Autodesk Inventor part; units mm, degrees
ref_plane "Work Plane19" through (16.25, 10, -160.125) normal (0, 0.3947, -0.9188) x (1, 0, 0)
ref_plane "Work Plane21" through (16.25, 10, -160.125) normal (0, 0.9118, 0.4107) x (1, 0, 0)
ref_plane "Work Plane22" through (16.25, 101.1762, -119.0531) normal (0, 0.9118, 0.4107) x (1, 0, 0)
sketch "Sketch1" plane through (0, 0, 0) normal (0, 1, 0) x (-1, 0, 0)
  circle A0 centre (0, 0) radius 135
  circle A1 centre (0, 0) radius 115
  circle A2 centre (0, 0) radius 112.0375
  circle A3 centre (0, 0) radius 9.5
  circle A4 centre (0, 0) radius 125
  circle A5 centre (0, -125) radius 2.75
  circle A6 centre (73.4732, -101.1271) radius 2.75
  circle A7 centre (118.8821, -38.6271) radius 2.75
  circle A8 centre (118.8821, 38.6271) radius 2.75
  circle A9 centre (73.4732, 101.1271) radius 2.75
  circle A10 centre (0, 125) radius 2.75
  circle A11 centre (-73.4732, 101.1271) radius 2.75
  circle A12 centre (-118.8821, 38.6271) radius 2.75
  circle A13 centre (-118.8821, -38.6271) radius 2.75
  circle A14 centre (-73.4732, -101.1271) radius 2.75
  dimension "d264" = 250
  dimension "Absolute_Diameter" = 270
  dimension "Diameter_No_Outer_Lip" = 230
  dimension "Inner_Cylinder_Diameter" = 224.075
  dimension "Lip_Diameter" = 19
  dimension "d265" = 5.5
  dimension "d268" = 360
extrude "Extrusion1" add sketch "Sketch1" along normal blind 10 contours A0 | A4 A7 A6 A5 A14 A13 A12 A11 A10 A9 A8
extrude "Extrusion2" add sketch "Sketch1" along normal blind 105.5 contours A1
sketch "Sketch2" plane through (0, 105.5, 0) normal (0, 1, 0) x (1, 0, 0)
  circle A0 centre (0, 0) radius 115
  circle A1 centre (0, 0) radius 68.375
  dimension "Lip_Diameter_Out" = 230
  dimension "Inner_Lip_Diameter" = 136.75
extrude "Extrusion7" add sketch "Sketch2" against normal blind 5
sketch "Sketch28" plane through (0, 10, 0) normal (0, 1, 0) x (1, 0, 0)
  line L0 (-77.5, -75) -> (77.5, -75)
  line L1 (77.5, -75) -> (77.5, -175)
  line L2 (77.5, -175) -> (-77.5, -175)
  line L3 (-77.5, -175) -> (-77.5, -75)
  circle A0 centre (0, -125) radius 2.75
  line L4 (-77.5, -75) -> (77.5, -175) construction
  line L5 (77.5, -75) -> (-77.5, -175) construction
  point P0 (0, 0)
  dimension "d271" = 155
  dimension "d272" = 100
extrude "Extrusion34" cut sketch "Sketch28" along normal up to surface (90.5 mm away)
sketch "Sketch30" plane through (0, 10, 0) normal (0, 1, 0) x (1, 0, 0)
  point P0 (0, 0)
ref_plane "Work Plane19" through (16.25, 10, -160.125) normal (0, 0.3947, -0.9188) x (1, 0, 0)
ref_plane "Work Plane21" through (16.25, 10, -160.125) normal (0, 0.9118, 0.4107) x (1, 0, 0)
ref_plane "Work Plane22" through (16.25, 101.1762, -119.0531) normal (0, 0.9118, 0.4107) x (1, 0, 0)
sketch "Sketch31" plane through (16.25, 101.1762, -119.0531) normal (0, 0.9118, 0.4107) x (1, 0, 0)
  circle A0 centre (-16.25, -239.1031) radius 20
  point P0 (-16.25, -150.1031)
  dimension "d286" = 40
  dimension "d289" = 89
extrude "Extrusion36" cut sketch "Sketch31" along normal mid plane 52.8625
fillet "Fillet19" radius 5 2 edges at (-77.5, 55.25, 80.9083) (77.5, 55.25, 80.9083)
properties part number "Cylinder Segment  Camera only"
CAD build for the part. Positions are in the model's coordinates, mm. A direction names the side the tool comes from. Round coordinates to 2 decimals unless told otherwise and drop trailing zeros. Loops run counter-clockwise (first coordinate to the right, second up) from the corner with the lowest first, then second, coordinate; pieces in that order, holes last. Notation, with made-up numbers: M 53.5,-21 L 99.5,-21 A20 ccw 99.5,2 Z; hole C 50,10 d10. An arc over 180 degrees is marked long. Use a Markdown table: item, result. Add a question column.
(1) Cut at B-B (x = -30). Give the cut face in (y, z), and give its area (3 significant figures).
(2) Which spindle directions (+Z, -Z, +X, -X, +Y, -Y) get a long thin tool onto all of the face, cutting with end or side? Do faces 4 (the face through (-4.7, 49.55, -111.94)), 5 (the face through (-50, 105.5, -50)). Say none if no direction does.
(3) Cut at C-C (y = 52.5). Give the cut face in (x, z) (1 decimal), and give its area (3 significant figures).
(4) Flat gauge pins, fed straight in: pin 1 (6 mm diameter, centred on x = 93.5, z = 41.5, fed in from -Y); pin 2 (3.5 mm diameter, centred on x = -73.47, z = 101.13, fed in from +Y); pin 3 (2 mm diameter, centred on y = 35, z = 84, fed in from -X); pin 4 (1.5 mm diameter, centred on x = -100, y = 52, fed in from +Z). Where does each tip first touch, or does it go through?
(5) Drill centre lines: line 1 (Z direction, x = 0, y = 6.5); line 2 (X direction, y = 64, z = 0); line 3 (Z direction, x = 0, y = 2). Where is each one in solid material? Low to high.
(6) Pull direction X, two halves, no side cores. Call faces 1 (the face through (51, 0, 101)), 2 (the face through (0.33, 3.257, 121.013)), 3 (the face through (14.97, 57.08, -114.02)): +X half, -X half, draft (parallel to the pull), parting line (faces both ways), or undercut.
(7) Cut at A-A (z = 0). Give the cut face in (x, y) (1 decimal), and give its area (3 significant figures).
(8) Cut at D-D (x = -106.5). Give the cut face in (y, z).
Geometry says:
| question | item | result |
|---|---|---|
| 1 | outline | M 0,-131.62 L 10,-131.62 L 10,-111.02 L 105.5,-111.02 L 105.5,-61.44 L 100.5,-61.44 L 100.5,-107.95 L 0,-107.95 Z; M 0,107.95 L 10,107.95 L 10,131.62 L 0,131.62 Z; M 100.5,61.44 L 105.5,61.44 L 105.5,111.02 L 100.5,111.02 Z |
| 1 | area | 1,250 mm² |
| 2 | face 4 | -Y |
| 2 | face 5 | +Z, -Z, +X, -X, +Y |
| 3 | outline | M -79,79.5 A5 ccw -77.5,83 L -77.5,85 A115 ccw long 77.5,85 L 77.5,83 A5 ccw 79,79.5 A112 cw long Z |
| 3 | area | 1,610 mm² |
| 4 | pin 1 | stops at y = 100.5 |
| 4 | pin 2 | passes through |
| 4 | pin 3 | stops at x = -79.6 |
| 4 | pin 4 | stops at z = 58.09 |
| 5 | line 1 | z = -135 to -127.75, -122.25 to -112.04, 127.75 to 135 |
| 5 | line 2 | x = -115 to -112.04, 112.04 to 115 |
| 5 | line 3 | z = -135 to -127.75, -122.25 to -112.04, 120.45 to 122.25, 127.75 to 135 |
| 6 | face 1 | draft |
| 6 | face 2 | undercut |
| 6 | face 3 | parting line |
| 7 | outline | M -135,0 L -112,0 L -112,100.5 L -68.4,100.5 L -68.4,105.5 L -115,105.5 L -115,10 L -135,10 Z; M 68.4,100.5 L 112,100.5 L 112,0 L 135,0 L 135,10 L 115,10 L 115,105.5 L 68.4,105.5 Z |
| 7 | area | 1,460 mm² |
| 8 | outline | M 0,-82.96 L 10,-82.96 L 10,-43.39 L 105.5,-43.39 L 105.5,43.39 L 10,43.39 L 10,82.96 L 0,82.96 L 0,34.79 L 100.5,34.79 L 100.5,-34.79 L 0,-34.79 Z |
